Design review of the part built by this model. Coordinates are the model's own, in mm. Coordinates: 2 decimals unless noted, no trailing zeros. Loops run counter-clockwise (first coordinate to the right, second up) from the corner with the lowest first, then second, coordinate; pieces in that order, holes last. Notation, with made-up numbers: (77, 10) -> (87, 10) arc R22 cw to (87, 20) -> close; hole circle Ø8 at (64, 49). An arc over 180 degrees is marked (long way). Answer in a Markdown table with one row per item.
Solid Edge part; units mm, degrees
sketch "Sketch1" plane through (0, 0, 0) normal (0, -1, 0) x (1, 0, 0)
  line L0 (-10.75, -7.5) -> (10.75, -7.5)
  line L1 (10.75, -7.5) -> (10.75, 7.5)
  line L2 (10.75, 7.5) -> (-10.75, 7.5)
  line L3 (-10.75, 7.5) -> (-10.75, -7.5)
  dimension "D1" = 10.75
  dimension "D2" = 10.75
extrude "Protrusion1" add sketch "Sketch1" against normal blind 50
hole "Hole_1" at (10.75, 15, 0) direction (-1, 0, 0) diameter 8.4 end up to next
hole "Hole1" at (10.75, 42.65, 0) direction (-1, 0, 0) diameter 8.4 end up to next
(1) Take a section at D-D on z = 0. Give the boundary of the cut face in (x, y).
Evaluation:
| item | result |
|---|---|
| outline | (-10.75, 0) -> (10.75, 0) -> (10.75, 10.8) -> (-10.75, 10.8) -> close; (-10.75, 19.2) -> (10.75, 19.2) -> (10.75, 38.45) -> (-10.75, 38.45) -> close; (-10.75, 46.85) -> (10.75, 46.85) -> (10.75, 50) -> (-10.75, 50) -> close |
(2) Take a section at A-A on y = 15. Give the boundary of the cut face in (x, z).
Evaluation:
| item | result |
|---|---|
| outline | (-10.75, -7.5) -> (10.75, -7.5) -> (10.75, -4.2) -> (-10.75, -4.2) -> close; (-10.75, 4.2) -> (10.75, 4.2) -> (10.75, 7.5) -> (-10.75, 7.5) -> close |
(3) Take a section at C-C on x = 0.25. Give the boundary of the cut face in (y, z).
Evaluation:
| item | result |
|---|---|
| outline | (0, -7.5) -> (50, -7.5) -> (50, 7.5) -> (0, 7.5) -> close; hole circle Ø8.4 at (15, 0); hole circle Ø8.4 at (42.65, 0) |
(4) Take a section at B-B on z = 2.5. Give the boundary of the cut face in (x, y).
Evaluation:
| item | result |
|---|---|
| outline | (-10.75, 0) -> (10.75, 0) -> (10.75, 11.63) -> (-10.75, 11.63) -> close; (-10.75, 18.37) -> (10.75, 18.37) -> (10.75, 39.28) -> (-10.75, 39.28) -> close; (-10.75, 46.02) -> (10.75, 46.02) -> (10.75, 50) -> (-10.75, 50) -> close |
(5) Draft analysis for pull direction Z (two halves, no side actions). For faces 1 (the flat face through (0, 0, 0)), 2 (the flat face through (0, 25, -7.5)), 3 (the cylindrical face through (0.15, 46.19, -2.26)), state which applies: pulls with the +Z half, pulls with the -Z half, needs draft (parallel to the pull), parting line crosses it, or undercut.
Evaluation:
| item | result |
|---|---|
| face 1 | needs draft |
| face 2 | pulls with the -Z half |
| face 3 | undercut |
(6) To check wall thickness, follow probe 1 along Y at (x, z) = (4, 0); probe 2 along Y at (x, z) = (4.75, -3); probe 3 along Z at (x, y) = (4.75, 42.65). State the ranges of each line that lie inside material, in increasing order.
Evaluation:
| item | result |
|---|---|
| probe 1 | y = 0 to 10.8, 19.2 to 38.45, 46.85 to 50 |
| probe 2 | y = 0 to 12.06, 17.94 to 39.71, 45.59 to 50 |
| probe 3 | z = -7.5 to -4.2, 4.2 to 7.5 |
